from build123d import *

# Parameters (mm, degrees)
SKETCH1_R               = 6
BOSS_EXTRUDE1_DEPTH     = 106
CHAMFER1_SIZE           = 0.5
CUT_EXTRUDE1_DEPTH      = 107.339080304
CUT_EXTRUDE1_DEPTH_BACK = 107.339080304
SKETCH2_R               = 1.5
SKETCH4_W               = 7.302801642
SKETCH4_H               = 16.597276459
CUT_EXTRUDE2_DEPTH      = 107.687628166


with BuildPart() as part:
    # Sketch1 → Boss-Extrude1 (new body)
    with BuildSketch(Plane(origin=(0, 0, 0), x_dir=(1, 0, 0), z_dir=(0, 1, 0))):
        with Locations(Location((0, 0, 0), (0, 0, 270))):
            Circle(SKETCH1_R)
    extrude(amount=BOSS_EXTRUDE1_DEPTH)

    # Chamfer1
    chamfer1_edges = [part.edges().sort_by_distance(p)[0] for p in [
        (0, 0, -6),
        (0, 106, -6),
    ]]
    chamfer(chamfer1_edges, length=CHAMFER1_SIZE)

    # Sketch2 → Cut-Extrude1 (cut, two sides: drawn at the far end of the back side and taken through both)
    with BuildSketch(Plane(origin=(0, 0, 0), x_dir=(0, 0, -1), z_dir=(1, 0, 0)).offset(-CUT_EXTRUDE1_DEPTH_BACK)):
        with Locations((0, 5)):
            Circle(SKETCH2_R)
    extrude(amount=CUT_EXTRUDE1_DEPTH + CUT_EXTRUDE1_DEPTH_BACK, mode=Mode.SUBTRACT)

    # Sketch4 → Cut-Extrude2 (cut, through all)
    with BuildSketch(Plane.XY.offset(4.5)):
        with Locations((0, 104.298638229)):
            Rectangle(SKETCH4_W, SKETCH4_H)
    extrude(amount=CUT_EXTRUDE2_DEPTH, mode=Mode.SUBTRACT)


solid = part.part
The listing builds one solid part. Answer for the finished solid, in the listing's coordinates (mm). Round coordinates to 2 decimals unless told otherwise and drop trailing zeros. Write each loop counter-clockwise with the first axis right and the second up, starting at its lowest first coordinate (ties: lowest second). Pieces come first, ordered by that corner, then holes. Notation, with made-up numbers: M -32.5,-36 L -2.5,-36 A14 ccw -2.5,-9 Z; hole C 3,88 d2. An arc over 180 degrees is marked long. Write each question's results on one line, items separated by ' | '. Start each with the question number.
(1) Each of these flat-tipped pins is pushed along its axis until it touches: P1, Ø2, axis at x = 1.5, y = 100, coming from the +Z side; P2, Ø1.6, axis at x = 2, z = 5.5, coming from the +Y side. Where does it stop, or does it pass through?
(2) Find the intervals of material crossed by line 1 (Y direction, x = 0.75, z = 0); line 2 (Z direction, x = -0.25, y = 5); line 3 (X direction, y = 48, z = 0.5), in increasing order.
(3) Determine the mould class of faces 1 (the flat face through (0, 101, 4.5)), 2 (the cylindrical face through (-0.08, 5.07, 1.5)), 3 (the cylindrical face through (0, 52, -6)) for opening direction X: +X half, -X half, draft (parallel to the pull), parting line (faces both ways), or undercut.
(4) The part is cut by section D-D, the plane y = 70. Write down the section's boundary in (x, z).
(5) The part is cut by section A-A, the plane z = 0. Write down the section's boundary in (x, y).
(6) The part is cut by section B-B, the plane x = 0. Write down the section's boundary in (y, z), and give its area (3 significant figures).
(7) The part is cut by section C-C, the plane y = 5. Write down the section's boundary in (x, z).
Worked answers:
1) P1: stops at z = 4.5 | P2: stops at y = 96
2) line 1: y = 0 to 3.5, 6.5 to 106 | line 2: z = -5.99 to -1.5, 1.5 to 5.99 | line 3: x = -5.98 to 5.98
3) face 1: undercut | face 2: draft | face 3: parting line
4) outline: C 0,0 d12
5) outline: M -6,0.5 L -5.5,0 L 5.5,0 L 6,0.5 L 6,3.5 L -6,3.5 Z; M -6,6.5 L 6,6.5 L 6,105.5 L 5.5,106 L -5.5,106 L -6,105.5 Z
6) outline: M 0,-5.5 L 0.5,-6 L 105.5,-6 L 106,-5.5 L 106,4.5 L 96,4.5 L 96,6 L 0.5,6 L 0,5.5 Z; hole C 5,0 d3 | area: 1,250 mm²
7) outline: M -5.81,-1.5 A6 ccw 5.81,-1.5 Z; M -5.81,1.5 L 5.81,1.5 A6 ccw Z
